Read the model definition and answer for the solid it produces. Units are mm, in the model's axes. Face numbers are marked on the shaded views. A direction names the side the tool comes from. Give positions to 0.01 mm unless a question says otherwise; leave off trailing zeros. Order: outer loops, then holes, each group sorted by start corner. A loop starts at its lowest first (then second) coordinate and runs counter-clockwise, first axis right, second up.
```python
from build123d import *

# Parameters (mm, degrees)
F1_DEPTH = 10
F2_R     = 3.96875
F3_DEPTH = 12.93749
F4_R     = 6.002975
F5_R     = 3.96875
F7_DEPTH = 22.93749
F8_DEPTH = 6.58749


# Not quite as in the source:
# - a fillet or chamfer is up to 0.001 mm smaller than in the source, because OpenCascade refuses the exact size


with BuildPart() as f1:
    # F0 (on Top) → F1 (new body)
    with BuildSketch(Plane.XY):
        Polygon((6.0029852, 0), (0, 0), (0, -43.0059592), (6.0029852, -43.0059592), (12.0059704, -43.0059592), (12.0059704, 0), align=None)
        with BuildLine():
            ThreePointArc((7.5029852, -37.002974), (7.0636453718, -38.0636341718), (6.0029852, -38.502974))
            ThreePointArc((6.0029852, -38.502974), (4.5029852, -37.002974), (6.0029852, -35.502974))
            ThreePointArc((6.0029852, -35.502974), (7.0636453718, -35.9423138282), (7.5029852, -37.002974))
        make_face(mode=Mode.SUBTRACT)
        with BuildLine():
            ThreePointArc((6.0029852, -7.5029852), (4.5029852, -6.0029852), (6.0029852, -4.5029852))
            ThreePointArc((6.0029852, -4.5029852), (7.0636453718, -4.9423250282), (7.5029852, -6.0029852))
            ThreePointArc((7.5029852, -6.0029852), (7.0636453718, -7.0636453718), (6.0029852, -7.5029852))
        make_face(mode=Mode.SUBTRACT)
    extrude(amount=F1_DEPTH)

    # F2 (on face) → F3 (join)
    with BuildSketch(Plane.XY.offset(10)):
        with BuildLine():
            Line((12.0059704, -43.0059592), (12.0059704, 0))
            Line((12.0059704, 0), (-3.96875, 0))
            Line((-3.96875, 0), (-3.96875, -1.68275))
            ThreePointArc((-3.96875, -1.68275), (-2.3523038982, -2.3523038982), (-1.68275, -3.96875))
            ThreePointArc((-1.68275, -3.96875), (-3.96875, -6.25475), (-6.25475, -3.96875))
            Line((-6.25475, -3.96875), (-7.9375, -3.96875))
            Line((-7.9375, -3.96875), (-7.9375, -43.0059592))
            Line((-7.9375, -43.0059592), (-3.96875, -43.0059592))
            Line((-3.96875, -43.0059592), (12.0059704, -43.0059592))
        make_face()
        with BuildLine():
            ThreePointArc((-1.68275, -39.0372092), (-2.3523038982, -40.6536553018), (-3.96875, -41.3232092))
            ThreePointArc((-3.96875, -41.3232092), (-5.5851961018, -37.4207630982), (-1.68275, -39.0372092))
        make_face(mode=Mode.SUBTRACT)
        with Locations((6.0029852, -37.002974)):
            Circle(F2_R, mode=Mode.SUBTRACT)
        with Locations((6.0029852, -6.0029852)):
            Circle(F2_R, mode=Mode.SUBTRACT)
        with BuildLine():
            Line((-3.96875, -1.68275), (-3.96875, 0))
            Line((-3.96875, 0), (-7.9375, 0))
            Line((-7.9375, 0), (-7.9375, -3.96875))
            Line((-7.9375, -3.96875), (-6.25475, -3.96875))
            ThreePointArc((-6.25475, -3.96875), (-5.5851961018, -2.3523038982), (-3.96875, -1.68275))
        make_face()
    extrude(amount=F3_DEPTH)

    # F4 (radius 6.0029852 in the source; OpenCascade refuses exactly that, so slightly less here)
    f4_edges = [f1.edges().sort_by_distance(p)[0] for p in [
        (12.00597, 0, 11.468745),
        (0, 0, 5),
        (0, -43.005959, 5),
        (12.00597, -43.005959, 11.468745),
    ]]
    fillet(f4_edges, radius=F4_R)

    # F5
    f5_edges = [f1.edges().sort_by_distance(p)[0] for p in [
        (-7.9375, -43.005959, 16.468745),
        (-7.9375, 0, 16.468745),
    ]]
    fillet(f5_edges, radius=F5_R)

    # F6 (on face) → F7 (cut, through all)
    with BuildSketch(Plane(origin=(0, 0, 0), x_dir=(1, 0, 0), z_dir=(0, 0, -1))):
        with BuildLine():
            ThreePointArc((12.0059704, 30.145029001), (9.5274974569, 26.1361174223), (8.6624922, 21.5029796))
            Line((8.6624922, 21.5029796), (12.0059704, 21.5029796))
            Line((12.0059704, 21.5029796), (12.0059704, 30.145029001))
        make_face()
        with BuildLine():
            Line((12.0059704, 21.5029796), (8.6624922, 21.5029796))
            ThreePointArc((8.6624922, 21.5029796), (9.5274974569, 16.8698417777), (12.0059704, 12.860930199))
            Line((12.0059704, 12.860930199), (12.0059704, 21.5029796))
        make_face()
    extrude(amount=-F7_DEPTH, mode=Mode.SUBTRACT)

    # F8 (cut): a face of the model
    f8_faces = [f1.faces().sort_by_distance(p)[0] for p in [
        (-3.6441940758, -21.5029796, 10),
    ]]
    extrude(f8_faces, amount=-F8_DEPTH, mode=Mode.SUBTRACT)


solid = f1.part
```
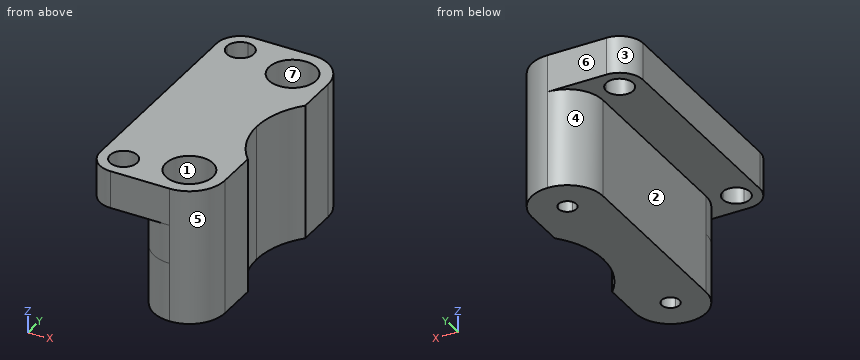
1) The part is cut by section A-A on z = 18.25. Determine the outline of the cut face in (x, y), and give its area (3 significant figures).
Final values:
outline: (-7.94, -39.04) arc R3.97 ccw to (-3.97, -43.01) - (6, -43.01) arc R6 ccw to (12.01, -37) - (12.01, -30.15) arc R12.84 cw to (12.01, -12.86) - (12.01, -6) arc R6 ccw to (6, 0) - (-3.97, 0) arc R3.97 ccw to (-7.94, -3.97) - close; hole circle Ø4.57 at (-3.97, -39.04); hole circle Ø4.57 at (-3.97, -3.97); hole circle Ø7.94 at (6, -37); hole circle Ø7.94 at (6, -6)
area: 664 mm2
2) A tool of negligible diameter and unlimited length cuts with its end or side. For the marked faces 1, 2, 3 and 4, from which of +Z, -Z, +X, -X, +Y, -Y can it reach the whole face along a straight path? Write none if from no direction.
Final values:
face 1: +Z
face 2: -Z, -X, +Y, -Y
face 3: +Z, -Z, -X, +Y
face 4: -Z, -X, +Y
3) Given pin 1 (7.5 mm diameter, centred on x = -3.97, y = -39.04, fed in from -Z); pin 2 (1 mm diameter, centred on y = -27.5, z = 11, fed in from +X); pin 3 (4 mm diameter, centred on x = 7, y = -5.5, fed in from +Z); pin 4 (1.5 mm diameter, centred on x = -1.5, z = 7, fed in from -Y), each flat-ended and moving along its own axis, determine where each tip first touches the part or whether it passes through.
Final values:
pin 1: stops at z = 16.59
pin 2: stops at x = 10.43
pin 3: stops at z = 10
pin 4: passes through
4) Consider L1, parallel to X at y = -37, z = 6.5; L2, parallel to Y at x = 8.25, z = 17; L3, parallel to Y at x = -4.75, z = 17.75. Determine where each line is inside the solid, lowest interval first.
Final values:
L1: x = 0 to 4.5, 7.5 to 12.01
L2: y = -42.57 to -40.27, -33.73 to -9.27, -2.73 to -0.44
L3: y = -42.93 to -41.19, -36.89 to -6.12, -1.82 to -0.08
5) The part is cut by section D-D on x = 6.75. Determine the outline of the cut face in (y, z).
Final values:
outline: (-42.96, 0) - (-38.3, 0) - (-38.3, 10) - (-40.9, 10) - (-40.9, 22.94) - (-42.96, 22.94) - close; (-35.7, 0) - (-7.3, 0) - (-7.3, 10) - (-9.9, 10) - (-9.9, 22.94) - (-33.11, 22.94) - (-33.11, 10) - (-35.7, 10) - close; (-4.7, 0) - (-0.05, 0) - (-0.05, 22.94) - (-2.11, 22.94) - (-2.11, 10) - (-4.7, 10) - close
6) For a pull along Y with two mould halves and no side action, classify the marked faces 5, 6 and 7 as released by +Y, released by -Y, zero draft, split by the parting line, or undercut.
Final values:
face 5: released by -Y
face 6: released by +Y
face 7: undercut
7) The part is cut by section C-C on y = -7. Determine the outline of the cut face in (x, z).
Final values:
outline: (-7.94, 16.59) - (0, 16.59) - (0, 0) - (4.88, 0) - (4.88, 10) - (2.16, 10) - (2.16, 22.94) - (-7.94, 22.94) - close; (7.12, 0) - (12.01, 0) - (12.01, 22.94) - (9.84, 22.94) - (9.84, 10) - (7.12, 10) - close
8) The part is cut by section B-B on z = 5. Count the separate pieces of the cut face and the enclosed holes in it, and give its area (3 significant figures).
Final values:
separate pieces: 1
enclosed holes: 2
area: 432 mm2
